Can you work these out from the model? Positions are in its coordinate system, mm. Face numbers are marked on the shaded views. A direction names the side the tool comes from. Coordinates: 2 decimals unless noted, no trailing zeros. Order: outer loops, then holes, each group sorted by start corner. A loop starts at its lowest first (then second) coordinate and runs counter-clockwise, first axis right, second up.
```python
from build123d import *

# Parameters (mm, degrees)
SKETCH1_R                = 23.525
SKETCH1_R_2              = 2
BOSS_EXTRUDE1_DEPTH      = 44
BOSS_EXTRUDE2_DEPTH      = 16
BOSS_EXTRUDE2_DEPTH_BACK = 16
SKETCH2_R                = 23.6
SKETCH2_R_2              = 20


with BuildPart() as part:
    # Sketch1 → Boss-Extrude1 (new body)
    with BuildSketch(Plane.XY):
        with BuildLine():
            Line((-16.5, -28), (16.5, -28))
            ThreePointArc((16.5, -28), (0, 32.5), (-16.5, -28))
        make_face()
        Circle(SKETCH1_R, mode=Mode.SUBTRACT)
        with Locations((0, 28)):
            Circle(SKETCH1_R_2, mode=Mode.SUBTRACT)
        with Locations((24.286071043, 13.978430346)):
            Circle(SKETCH1_R_2, mode=Mode.SUBTRACT)
        with Locations((24.286071043, -14.064708963)):
            Circle(SKETCH1_R_2, mode=Mode.SUBTRACT)
        with Locations((-24.286071043, -14.064708963)):
            Circle(SKETCH1_R_2, mode=Mode.SUBTRACT)
        with Locations((-24.286071043, 13.978430346)):
            Circle(SKETCH1_R_2, mode=Mode.SUBTRACT)
    extrude(amount=BOSS_EXTRUDE1_DEPTH)

    # Sketch2 → Boss-Extrude2 (add, two sides: drawn at the far end of the back side and taken through both)
    with BuildSketch(Plane.XY.offset(22).offset(-BOSS_EXTRUDE2_DEPTH_BACK)):
        Circle(SKETCH2_R)
        Circle(SKETCH2_R_2, mode=Mode.SUBTRACT)
    extrude(amount=BOSS_EXTRUDE2_DEPTH + BOSS_EXTRUDE2_DEPTH_BACK)


solid = part.part
```
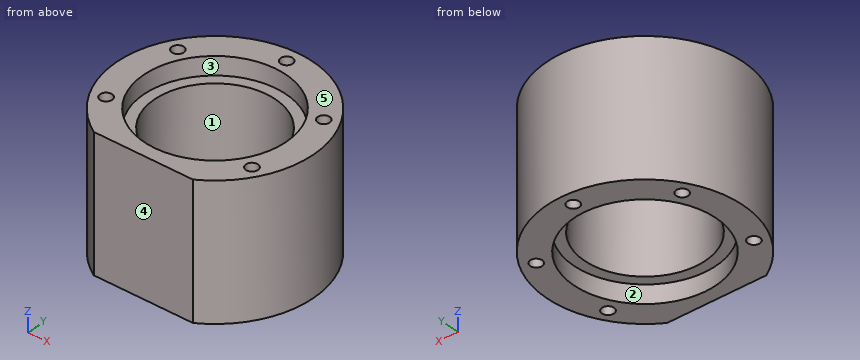
1. Please list where these lines run through material, in increasing order: probe 1 along Y at (x, z) = (-26, 37); probe 2 along Y at (x, z) = (12.5, 7); probe 3 along Z at (x, y) = (-21, -4).
Completed:
probe 1: y = -19.5 to -15.1, -13.03 to 12.95, 15.01 to 19.5
probe 2: y = -28 to -15.61, 15.61 to 30
probe 3: z = 6 to 38
2. Thinking about a two-plate mould opening in Y: for the marked faces 3, 4 and 5, which applies, pulls with the +Y half, pulls with the -Y half, needs draft (parallel to the pull), parting line crosses it, or undercut?
Completed:
face 3: undercut
face 4: pulls with the -Y half
face 5: needs draft
3. Imagine slicing it at A-A on y = 0. Please give me the cut outline in (x, z) (3 decimals).
Completed:
outline: (-32.5, 0) - (-23.525, 0) - (-23.525, 6) - (-20, 6) - (-20, 38) - (-23.525, 38) - (-23.525, 44) - (-32.5, 44) - close; (20, 6) - (23.525, 6) - (23.525, 0) - (32.5, 0) - (32.5, 44) - (23.525, 44) - (23.525, 38) - (20, 38) - close
4. Imagine slicing it at D-D on z = 23. Please give me the cut outline in (x, y), then the cut area to 3 significant figures.
Completed:
outline: (-16.5, -28) - (16.5, -28) arc R32.5 ccw (long way) to start; hole circle Ø4 at (-24.29, -14.06); hole circle Ø4 at (-24.29, 13.98); hole circle Ø40 at (0, 0); hole circle Ø4 at (0, 28); hole circle Ø4 at (24.29, -14.06); hole circle Ø4 at (24.29, 13.98)
area: 1,900 mm2
5. On a 3-axis mill with a long thin cutter (end or side, diameter ignored), from which of +Z, -Z, +X, -X, +Y, -Y can I reach the whole of each face in a straight line? I mean the marked faces 1 and 2. Say none if no direction works.
Completed:
face 1: +Z, -Z
face 2: -Z
6. Imagine slicing it at C-C on x = 7.5. Please give me the cut outline in (y, z).
Completed:
outline: (-28, 0) - (-22.3, 0) - (-22.3, 6) - (-18.54, 6) - (-18.54, 38) - (-22.3, 38) - (-22.3, 44) - (-28, 44) - close; (18.54, 6) - (22.3, 6) - (22.3, 0) - (31.62, 0) - (31.62, 44) - (22.3, 44) - (22.3, 38) - (18.54, 38) - close
7. I'm going to push flat-ended pins straight in: pin 1 (3 mm diameter, centred on x = 24.29, y = 13.98, fed in from +Z); pin 2 (1.5 mm diameter, centred on x = -19.5, y = -10.5, fed in from -Z); pin 3 (8 mm diameter, centred on y = 21, z = 16.5, fed in from +X); pin 4 (1 mm diameter, centred on x = -8.5, z = 10.5, fed in from +Y). Where does each tip first touch, or does it pass through?
Completed:
pin 1: passes through
pin 2: stops at z = 6
pin 3: stops at x = 27.7
pin 4: stops at y = 31.5
8. Imagine slicing it at B-B on x = 0. Please give me the cut outline in (y, z) (3 decimals).
Completed:
outline: (-28, 0) - (-23.525, 0) - (-23.525, 6) - (-20, 6) - (-20, 38) - (-23.525, 38) - (-23.525, 44) - (-28, 44) - close; (20, 6) - (23.525, 6) - (23.525, 0) - (26, 0) - (26, 44) - (23.525, 44) - (23.525, 38) - (20, 38) - close; (30, 0) - (32.5, 0) - (32.5, 44) - (30, 44) - close
